```python
from build123d import *

# Parameters (mm, degrees)
F0_R     = 17.2
F1_DEPTH = 30
F2_R     = 16.65
F3_DEPTH = 22
F4_R     = 13.2
F5_DEPTH = 25
F6_R     = 13.2
F7_DEPTH = 30


with BuildPart() as f1:
    # F0 (on Top) → F1 (new body)
    with BuildSketch(Plane.XY):
        Circle(F0_R)
    extrude(amount=F1_DEPTH)

    # F2 (on face) → F3 (join)
    with BuildSketch(Plane.XY.offset(30)):
        Circle(F2_R)
    extrude(amount=F3_DEPTH)

    # F4 (on face) → F5 (cut)
    with BuildSketch(Plane.XY.offset(52)):
        Circle(F4_R)
    extrude(amount=-F5_DEPTH, mode=Mode.SUBTRACT)

    # F6 (on face) → F7 (cut)
    with BuildSketch(Plane(origin=(0, 0, 0), x_dir=(1, 0, 0), z_dir=(0, 0, -1))):
        Circle(F6_R)
    extrude(amount=-F7_DEPTH, mode=Mode.SUBTRACT)


solid = f1.part
```
Can you work these out from the model? Positions are in its coordinate system, mm. A direction names the side the tool comes from. Round coordinates to 2 decimals unless told otherwise and drop trailing zeros. Loops run counter-clockwise (first coordinate to the right, second up) from the corner with the lowest first, then second, coordinate; pieces in that order, holes last. Notation, with made-up numbers: M 69,52 L 111,52 A28 ccw 111,85 Z; hole C -22.5,45.5 d6. An arc over 180 degrees is marked long. Answer in a Markdown table with one row per item.
1. I'm going to push flat-ended pins straight in: pin 1 Ø1 at (x, z) = (6.5, 32.5) entering from +Y; pin 2 Ø4 at (y, z) = (9.5, 25) entering from +X; pin 3 Ø12 at (x, z) = (-10, 29.5) entering from -Y. Where does each tip first touch, or does it pass through?
Established:
| item | result |
|---|---|
| pin 1 | y = 15.53 |
| pin 2 | x = 15.48 |
| pin 3 | y = -16.73 |
2. If we section it at C-C, the plane z = 25: Please give me the cut outline in (x, y), plus the area to 3 significant figures.
Established:
| item | result |
|---|---|
| outline | C 0,0 d34.4; hole C 0,0 d26.4 |
| area | 382 mm² |
3. If we section it at D-D, the plane z = 48.5: Please give me the cut outline in (x, y), plus the area to 3 significant figures.
Established:
| item | result |
|---|---|
| outline | C 0,0 d33.3; hole C 0,0 d26.4 |
| area | 324 mm² |
4. If we section it at A-A, the plane y = 0: Please give me the cut outline in (x, z).
Established:
| item | result |
|---|---|
| outline | M -17.2,0 L -13.2,0 L -13.2,52 L -16.65,52 L -16.65,30 L -17.2,30 Z; M 13.2,0 L 17.2,0 L 17.2,30 L 16.65,30 L 16.65,52 L 13.2,52 Z |
5. Thinking about a two-plate mould opening in X: for faces 3 (the face through (-17.183, 0.756, 14.79)), 4 (the face through (-9.73, -8.92, 25.64)), 5 (the face through (-1, 17, 30)), which applies, pulls with the +X half, pulls with the -X half, needs draft (parallel to the pull), parting line crosses it, or undercut?
Established:
| item | result |
|---|---|
| face 3 | parting line crosses it |
| face 4 | undercut |
| face 5 | needs draft |
6. On a 3-axis mill with a long thin cutter (end or side, diameter ignored), from which of +Z, -Z, +X, -X, +Y, -Y can I reach the whole of each face in a straight line? I mean faces 1 (the face through (-10, 9, 52)), 2 (the face through (7.683, -14.771, 40.846)). Say none if no direction works.
Established:
| item | result |
|---|---|
| face 1 | +Z, +X, -X, +Y, -Y |
| face 2 | +Z |
7. Please list where these lines run through material, in increasing order: line 1 (Y direction, x = 0, z = 22); line 2 (Y direction, x = 0, z = 36); line 3 (X direction, y = 4, z = 26.5). Write a range as from..to.
Established:
| item | result |
|---|---|
| line 1 | -17.2..-13.2, 13.2..17.2 |
| line 2 | -16.65..-13.2, 13.2..16.65 |
| line 3 | -16.73..-12.58, 12.58..16.73 |
